Check sheet for the modelled part. Datum: model origin and axes. Units: mm. A direction names the side the tool comes from. Round coordinates to 2 decimals unless told otherwise and drop trailing zeros. Loops run counter-clockwise (first coordinate to the right, second up) from the corner with the lowest first, then second, coordinate; pieces in that order, holes last. Notation, with made-up numbers: (-37.75, -13) - (-10.75, -13) arc R30 cw to (-10.75, 23) - close; hole circle Ø6 at (72, -18). An arc over 180 degrees is marked (long way). Answer in a Markdown table with one row per item. Add a question column.
(1) Cross-section at A-A on x = 0. Enter the section's corners in (y, z).
(2) Cross-section at C-C on y = -2.5. Enter the section's corners in (x, z).
(3) Cross-section at D-D on z = -7.5. Enter the section's corners in (x, y).
(4) Access from +Z, -Z, +X, -X, +Y, -Y to the whole of each face (thin tool, end or side, straight path). Record for faces 4 (the flat face through (0, -13, -5)), 5 (the flat face through (3, -13, -8)), 6 (the flat face through (-3, -13, -8)), 7 (the flat face through (-0.95, -21, -8)), 8 (the flat face through (-5, 7, -0.4)).
(5) Cross-section at B-B on z = 8.5. Enter the section's corners in (x, y).
(6) Thickness scan on line 1 along Z through (x, y) = (-7.75, 14); line 2 along X through (y, z) = (12, 2.5); line 3 along X through (y, z) = (12, -10.5). Record the ranges inside material, lowest first.
(7) Mould release check, pull along Y, two halves, no side actions. Record for faces 1 (the flat face through (-0.65, -22.5, -8.5)), 2 (the flat face through (-7, 15, 0)), 3 (the flat face through (-5, 7, 0.4)): +Y half, -Y half, draft (parallel to the pull), parting line (faces both ways), or undercut.
(8) Gauge pin test, flat ends, axial feed: pin 1 (3 mm diameter, centred on x = 0, y = -6.5, fed in from -Z); pin 2 (1.5 mm diameter, centred on x = -6.5, z = 5, fed in from -Y); pin 3 (1.3 mm diameter, centred on y = -19.5, z = -10, fed in from +X). Record the tip position at first contact, or that the pin passes through.
from build123d import *
from build123d.topology import SkipClean

# Parameters (mm, degrees)
SKETCH_1_R               = 12
EXTRUDE_1_DEPTH          = 20
SKETCH_2_R               = 1.975
CUT_EXTRUDE_1_DEPTH      = 15
SKETCH_3_R               = 3
CUT_EXTRUDE_2_DEPTH      = 27.229754097
EXTRUDE_START            = 25
SKETCH_4_W               = 6
SKETCH_4_H               = 6.618950039
EXTRUDE_2_DEPTH          = 25
CUT_EXTRUDE_START        = -37
SKETCH_5_W               = 3.5
SKETCH_5_H               = 1.5
CUT_EXTRUDE_3_DEPTH      = 37
CUT_EXTRUDE_4_DEPTH      = 33.526911935
CUT_EXTRUDE_4_DEPTH_BACK = 5
SKETCH_6_W               = 1.3
SKETCH_6_H               = 4.2
SKETCH_7_W               = 1.3
SKETCH_7_H               = 5.2
CUT_EXTRUDE_5_DEPTH      = 36.397740041
SKETCH_8_W               = 1.9
SKETCH_8_H               = 2
CUT_EXTRUDE_6_DEPTH      = 33.526911935
CHAMFER_1_SIZE           = 0.5
SKETCH_9_W               = 1
SKETCH_9_H               = 0.8
CUT_EXTRUDE_7_DEPTH      = 15
PATTERN_CIRCULAR_1_COUNT = 8
MIRROR_1_COPY_1_SKETCH_W = 1
MIRROR_1_COPY_1_SKETCH_H = 0.8
MIRROR_1_COPY_1_DEPTH    = 15
MIRROR_1_COPY_2_SKETCH_W = 1
MIRROR_1_COPY_2_SKETCH_H = 0.8
MIRROR_1_COPY_2_DEPTH    = 15
MIRROR_1_COPY_3_SKETCH_W = 1
MIRROR_1_COPY_3_SKETCH_H = 0.8
MIRROR_1_COPY_3_DEPTH    = 15
MIRROR_1_COPY_4_SKETCH_W = 1
MIRROR_1_COPY_4_SKETCH_H = 0.8
MIRROR_1_COPY_4_DEPTH    = 15
MIRROR_1_COPY_5_SKETCH_W = 1
MIRROR_1_COPY_5_SKETCH_H = 0.8
MIRROR_1_COPY_5_DEPTH    = 15
MIRROR_1_COPY_6_SKETCH_W = 1
MIRROR_1_COPY_6_SKETCH_H = 0.8
MIRROR_1_COPY_6_DEPTH    = 15
MIRROR_1_COPY_7_SKETCH_W = 1
MIRROR_1_COPY_7_SKETCH_H = 0.8
MIRROR_1_COPY_7_DEPTH    = 15


with BuildPart() as part:
    # 草图1 → 凸台-拉伸1 (new body)
    with BuildSketch(Plane(origin=(0, 0, 0), x_dir=(1, 0, 0), z_dir=(0, 1, 0))):
        with Locations(Location((0, 0, 0), (0, 0, 270))):
            Circle(SKETCH_1_R)
    extrude(amount=EXTRUDE_1_DEPTH)

    # 草图2 → 切除-拉伸1 (cut)
    with BuildSketch(Plane.XZ):
        with Locations(Location((7.5, 0, 0), (0, 0, 270))):
            Circle(SKETCH_2_R)
        with Locations(Location((-7.5, 0, 0), (0, 0, 90))):
            Circle(SKETCH_2_R)
    extrude(amount=-CUT_EXTRUDE_1_DEPTH, mode=Mode.SUBTRACT)

    # 草图3 → 切除-拉伸2 (cut, through all)
    with BuildSketch(Plane.XZ):
        with Locations(Location((0, 8.5, 0), (0, 0, 270))):
            Circle(SKETCH_3_R)
    extrude(amount=-CUT_EXTRUDE_2_DEPTH, mode=Mode.SUBTRACT)

    # 草图4 → 凸台-拉伸2 (add)
    with SkipClean():  # the faces are left unmerged after this step: merging them gives an invalid solid
        with BuildSketch(Plane.XZ.offset(EXTRUDE_START)):
            with Locations((0, -8.30947502)):
                Rectangle(SKETCH_4_W, SKETCH_4_H)
            with BuildLine():
                Line((3, -11.618950039), (-3, -11.618950039))
                ThreePointArc((-3, -11.618950039), (0, -12), (3, -11.618950039))
            make_face()
        extrude(amount=-EXTRUDE_2_DEPTH)

    # 草图5 → 切除-拉伸3 (cut)
    with SkipClean():  # the faces are left unmerged after this step: merging them gives an invalid solid
        with BuildSketch(Plane(origin=(0, 20, 0), x_dir=(1, 0, 0), z_dir=(0, 1, 0)).offset(CUT_EXTRUDE_START)):
            with Locations((0, 11.121710071)):
                Rectangle(SKETCH_5_W, SKETCH_5_H)
            with BuildLine():
                Line((-1.75, 11.871710071), (1.75, 11.871710071))
                ThreePointArc((1.75, 11.871710071), (0, 12), (-1.75, 11.871710071))
            make_face()
        extrude(amount=CUT_EXTRUDE_3_DEPTH, mode=Mode.SUBTRACT)

    # 草图6 → 切除-拉伸4 (cut, two sides: drawn at the far end of the back side and taken through both)
    with SkipClean():  # the faces are left unmerged after this step: merging them gives an invalid solid
        with BuildSketch(Plane.XY.offset(-5).offset(-CUT_EXTRUDE_4_DEPTH_BACK)):
            with Locations((0, -20.9)):
                Rectangle(SKETCH_6_W, SKETCH_6_H)
        extrude(amount=CUT_EXTRUDE_4_DEPTH + CUT_EXTRUDE_4_DEPTH_BACK, mode=Mode.SUBTRACT)

    # 草图7 → 切除-拉伸5 (cut, through all)
    with SkipClean():  # the faces are left unmerged after this step: merging them gives an invalid solid
        with BuildSketch(Plane.XY.offset(-10)):
            with Locations((0, -20.9)):
                Rectangle(SKETCH_7_W, SKETCH_7_H)
        extrude(amount=-CUT_EXTRUDE_5_DEPTH, mode=Mode.SUBTRACT)

    # 草图8 → 切除-拉伸6 (cut, through all)
    with SkipClean():  # the faces are left unmerged after this step: merging them gives an invalid solid
        with BuildSketch(Plane.XY.offset(-5)):
            with Locations((0, -20.9)):
                Rectangle(SKETCH_8_W, SKETCH_8_H)
        extrude(amount=-CUT_EXTRUDE_6_DEPTH, mode=Mode.SUBTRACT)

    # 倒角1
    chamfer_1_edges = [part.edges().sort_by_distance(p)[0] for p in [
        (7.5, 0, 1.975),
        (-7.5, 0, -1.975),
    ]]
    chamfer(chamfer_1_edges, length=CHAMFER_1_SIZE)

    # 草图9 → 切除-拉伸7 (cut)
    with SkipClean():  # the faces are left unmerged after this step: merging them gives an invalid solid
        with BuildSketch(Plane.XZ):
            with Locations((5.065930456, 0)):
                Rectangle(SKETCH_9_W, SKETCH_9_H)
        cut_extrude_7 = extrude(amount=-CUT_EXTRUDE_7_DEPTH, mode=Mode.SUBTRACT)

    # 阵列(圆周)1: 切除-拉伸7 ×8 about axis
    with SkipClean():  # the faces are left unmerged after this step: merging them gives an invalid solid
        pattern_circular_1_axis = Axis((7.5, 0, 0), (0, 1, 0))
        for i in range(1, PATTERN_CIRCULAR_1_COUNT):
            add(cut_extrude_7.rotate(pattern_circular_1_axis, i * 360 / PATTERN_CIRCULAR_1_COUNT), mode=Mode.SUBTRACT)

    # 镜向1: 切除-拉伸7 across plane
    with SkipClean():  # the faces are left unmerged after this step: merging them gives an invalid solid
        add(cut_extrude_7.mirror(Plane(origin=(0, 0, 0), x_dir=(0, 0, 1), z_dir=(1, 0, 0))), mode=Mode.SUBTRACT)

    # 镜向1 copy 1 sketch → 镜向1 copy 1 (cut)
    with SkipClean():  # the faces are left unmerged after this step: merging them gives an invalid solid
        with BuildSketch(Plane(origin=(-2.196699141, 0, 5.303300859), x_dir=(-0.7071067811865476, 0, -0.7071067811865475), z_dir=(0, -1, 0))):
            with Locations((5.065930456, 0)):
                Rectangle(MIRROR_1_COPY_1_SKETCH_W, MIRROR_1_COPY_1_SKETCH_H)
        extrude(amount=-MIRROR_1_COPY_1_DEPTH, mode=Mode.SUBTRACT)

    # 镜向1 copy 2 sketch → 镜向1 copy 2 (cut)
    with SkipClean():  # the faces are left unmerged after this step: merging them gives an invalid solid
        with BuildSketch(Plane(origin=(-7.5, 0, 7.5), x_dir=(0, 0, -1), z_dir=(0, -1, 0))):
            with Locations((5.065930456, 0)):
                Rectangle(MIRROR_1_COPY_2_SKETCH_W, MIRROR_1_COPY_2_SKETCH_H)
        extrude(amount=-MIRROR_1_COPY_2_DEPTH, mode=Mode.SUBTRACT)

    # 镜向1 copy 3 sketch → 镜向1 copy 3 (cut)
    with SkipClean():  # the faces are left unmerged after this step: merging them gives an invalid solid
        with BuildSketch(Plane(origin=(-12.803300859, 0, 5.303300859), x_dir=(0.7071067811865475, 0, -0.7071067811865476), z_dir=(0, -1, 0))):
            with Locations((5.065930456, 0)):
                Rectangle(MIRROR_1_COPY_3_SKETCH_W, MIRROR_1_COPY_3_SKETCH_H)
        extrude(amount=-MIRROR_1_COPY_3_DEPTH, mode=Mode.SUBTRACT)

    # 镜向1 copy 4 sketch → 镜向1 copy 4 (cut)
    with SkipClean():  # the faces are left unmerged after this step: merging them gives an invalid solid
        with BuildSketch(Plane(origin=(-15, 0, 0), x_dir=(1, 0, 0), z_dir=(0, -1, 0))):
            with Locations((5.065930456, 0)):
                Rectangle(MIRROR_1_COPY_4_SKETCH_W, MIRROR_1_COPY_4_SKETCH_H)
        extrude(amount=-MIRROR_1_COPY_4_DEPTH, mode=Mode.SUBTRACT)

    # 镜向1 copy 5 sketch → 镜向1 copy 5 (cut)
    with SkipClean():  # the faces are left unmerged after this step: merging them gives an invalid solid
        with BuildSketch(Plane(origin=(-12.803300859, 0, -5.303300859), x_dir=(0.7071067811865477, 0, 0.7071067811865475), z_dir=(0, -1, 0))):
            with Locations((5.065930456, 0)):
                Rectangle(MIRROR_1_COPY_5_SKETCH_W, MIRROR_1_COPY_5_SKETCH_H)
        extrude(amount=-MIRROR_1_COPY_5_DEPTH, mode=Mode.SUBTRACT)

    # 镜向1 copy 6 sketch → 镜向1 copy 6 (cut)
    with SkipClean():  # the faces are left unmerged after this step: merging them gives an invalid solid
        with BuildSketch(Plane(origin=(-7.5, 0, -7.5), x_dir=(0, 0, 1), z_dir=(0, -1, 0))):
            with Locations((5.065930456, 0)):
                Rectangle(MIRROR_1_COPY_6_SKETCH_W, MIRROR_1_COPY_6_SKETCH_H)
        extrude(amount=-MIRROR_1_COPY_6_DEPTH, mode=Mode.SUBTRACT)

    # 镜向1 copy 7 sketch → 镜向1 copy 7 (cut)
    with SkipClean():  # the faces are left unmerged after this step: merging them gives an invalid solid
        with BuildSketch(Plane(origin=(-2.196699141, 0, -5.303300859), x_dir=(-0.7071067811865474, 0, 0.7071067811865477), z_dir=(0, -1, 0))):
            with Locations((5.065930456, 0)):
                Rectangle(MIRROR_1_COPY_7_SKETCH_W, MIRROR_1_COPY_7_SKETCH_H)
        extrude(amount=-MIRROR_1_COPY_7_DEPTH, mode=Mode.SUBTRACT)


solid = part.part
Answers:
| question | item | result |
|---|---|---|
| 1 | outline | (-25, -12) - (-23.5, -12) - (-23.5, -10) - (-23, -10) - (-23, -5) - (-25, -5) - close; (-18.8, -10) - (-18.3, -10) - (-18.3, -12) - (-17, -12) - (-17, -10.37) - (20, -10.37) - (20, 5.5) - (0, 5.5) - (0, -5) - (-18.8, -5) - close; (0, 11.5) - (20, 11.5) - (20, 12) - (0, 12) - close |
| 2 | outline | (-3, -11.62) arc R12 ccw to (-1.75, -11.87) - (-1.75, -10.37) - (1.75, -10.37) - (1.75, -11.87) arc R12 ccw to (3, -11.62) - (3, -5) - (-3, -5) - close |
| 3 | outline | (-9.37, 0) - (-3, 0) - (-3, -25) - (3, -25) - (3, 0) - (9.37, 0) - (9.37, 20) - (-9.37, 20) - close; hole (-0.95, -21.9) - (-0.65, -21.9) - (-0.65, -23) - (0.65, -23) - (0.65, -21.9) - (0.95, -21.9) - (0.95, -19.9) - (0.65, -19.9) - (0.65, -18.8) - (-0.65, -18.8) - (-0.65, -19.9) - (-0.95, -19.9) - close |
| 4 | face 4 | +Z, +X, -X, -Y |
| 4 | face 5 | +Z, -Z, +X, -Y |
| 4 | face 6 | +Z, -Z, -X, -Y |
| 4 | face 7 | +Z, -Z |
| 4 | face 8 | -Y |
| 5 | outline | (-8.47, 0) - (-3, 0) - (-3, 20) - (-8.47, 20) - close; (3, 0) - (8.47, 0) - (8.47, 20) - (3, 20) - close |
| 6 | line 1 | z = -9.16 to -2.93, 2.93 to 9.16 |
| 6 | line 2 | x = -11.74 to -7.9, -7.1 to 7.1, 7.9 to 11.74 |
| 6 | line 3 | x = -5.81 to -1.75, 1.75 to 5.81 |
| 7 | face 1 | undercut |
| 7 | face 2 | -Y half |
| 7 | face 3 | draft |
| 8 | pin 1 | stops at z = -10.37 |
| 8 | pin 2 | stops at y = 0 |
| 8 | pin 3 | stops at x = 3 |
